The figure shows three views and two pictorial views of one solid part (mm, origin at its lowest corner). Answer the questions. Give positions to 0.01 mm unless a question says otherwise; leave off trailing zeros. Order: outer loops, then holes, each group sorted by start corner. A loop starts at its lowest first (then second) coordinate and runs counter-clockwise, first axis right, second up. Notation, with made-up numbers: M 88,-11.75 L 147,-11.75 A29 cw 147,11.25 Z; hole C -22.5,18 d1. An arc over 180 degrees is marked long. Answer as a JSON object with one key per item and string values. Group by question number.
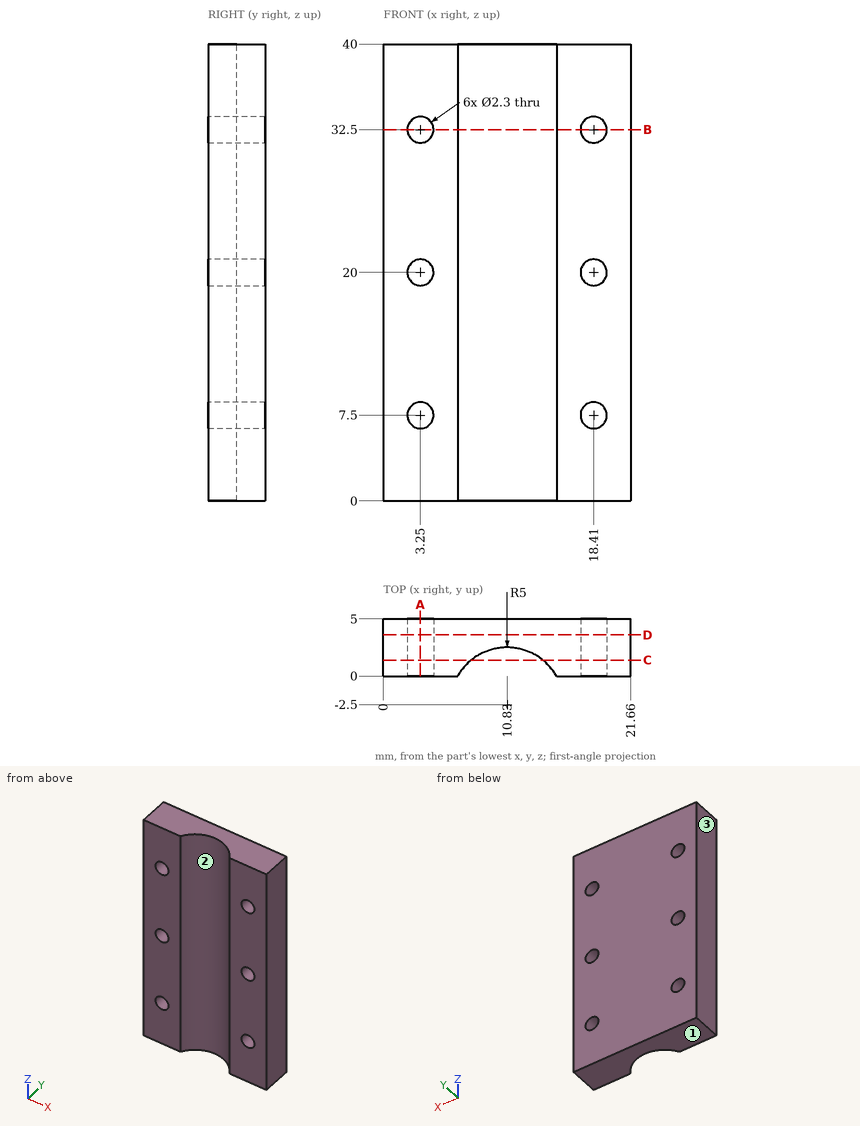
Item 1: Consider probe 1 along X at (y, z) = (3.55, 32.5); probe 2 along Z at (x, y) = (18.5, 1.2); probe 3 along X at (y, z) = (1.95, 32.5). Determine where each line is inside the solid, lowest interval first. Write a range as from..to.
Item 2: Section D-D (y = 3.6) is taken. Determine the outline of the cut face in (x, z).
Item 3: Section A-A (x = 3.25) is taken. Determine the outline of the cut face in (y, z).
Item 4: Section B-B (z = 32.5) is taken. Determine the outline of the cut face in (x, y).
Item 5: Determine the mould class of the marked faces 1, 2 and 3 for opening direction X: released by +X, released by -X, zero draft, split by the parting line, or undercut.
Item 6: Flat-ended cylindrical pins translate along their axes: P1, Ø3, axis at x = 18.41, z = 32.5, coming from the -Y side; P2, Ø1.4, axis at x = 3.25, z = 32.5, coming from the +Y side; P3, Ø6, axis at x = 10, z = 16.5, coming from the -Y side (1 decimal). Find the tip coordinate at first contact, or state that the pin passes through.
Item 7: Section C-C (y = 1.4) is taken. Determine the outline of the cut face in (x, z).
Values found:
{
 "1": {"probe 1": "x = 0..2.1, 4.4..17.26, 19.56..21.66", "probe 2": "z = 0..6.35, 8.65..18.85, 21.15..31.35, 33.65..40", "probe 3": "x = 0..2.1, 4.4..8.55, 13.11..17.26, 19.56..21.66"},
 "2": {"outline": "M 0,0 L 21.66,0 L 21.66,40 L 0,40 Z; hole C 3.25,7.5 d2.3; hole C 3.25,20 d2.3; hole C 3.25,32.5 d2.3; hole C 18.41,7.5 d2.3; hole C 18.41,20 d2.3; hole C 18.41,32.5 d2.3"},
 "3": {"outline": "M 0,0 L 5,0 L 5,6.35 L 0,6.35 Z; M 0,8.65 L 5,8.65 L 5,18.85 L 0,18.85 Z; M 0,21.15 L 5,21.15 L 5,31.35 L 0,31.35 Z; M 0,33.65 L 5,33.65 L 5,40 L 0,40 Z"},
 "4": {"outline": "M 0,0 L 2.1,0 L 2.1,5 L 0,5 Z; M 4.4,0 L 6.5,0 A5 cw 15.16,0 L 17.26,0 L 17.26,5 L 4.4,5 Z; M 19.56,0 L 21.66,0 L 21.66,5 L 19.56,5 Z"},
 "5": {"face 1": "zero draft", "face 2": "undercut", "face 3": "released by -X"},
 "6": {"P1": "stops at y = 0", "P2": "passes through", "P3": "stops at y = 0.7"},
 "7": {"outline": "M 0,0 L 7.7,0 L 7.7,40 L 0,40 Z; M 13.96,0 L 21.66,0 L 21.66,40 L 13.96,40 Z; hole C 3.25,7.5 d2.3; hole C 3.25,20 d2.3; hole C 3.25,32.5 d2.3; hole C 18.41,7.5 d2.3; hole C 18.41,20 d2.3; hole C 18.41,32.5 d2.3"}
}
